```python
from build123d import *

# Parameters (mm, degrees)
MAIN_EXTRUSION_DEPTH    = 4
CORNER_LEAVE_R          = 5
D_GAGEMENT_M41_D        = 4.5
ESQUISSE4_W             = 22
ESQUISSE4_H             = 72
ENL_V_MAT_EXTRU_1_DEPTH = 4
ENL_V_MAT_EXTRU_2_DEPTH = 4
CONG_1_R                = 4


with BuildPart() as part:
    # Main scetch → Main extrusion (new body)
    with BuildSketch(Plane(origin=(0, 0, 0), x_dir=(1, 0, 0), z_dir=(0, 1, 0))):
        Polygon((-150, 0), (150, 0), (150, 175), (105, 220), (-105, 220), (-150, 175), align=None)
    extrude(amount=MAIN_EXTRUSION_DEPTH)

    # Corner leave
    corner_leave_edges = [part.edges().sort_by_distance(p)[0] for p in [
        (150, 2, 0),
        (-150, 2, 0),
        (-150, 2, -175),
        (-105, 2, -220),
        (105, 2, -220),
        (150, 2, -175),
    ]]
    fillet(corner_leave_edges, radius=CORNER_LEAVE_R)

    # Dégagement M41 (through all)
    with Locations(Plane(origin=(0, 4, 0), x_dir=(1, 0, 0), z_dir=(0, 1, 0))):
        with Locations((-142, 8), (-142, 170), (142, 170), (142, 8), (0, 8)):
            Hole(D_GAGEMENT_M41_D / 2)

    # Esquisse4 → Enlèv. mat.-Extru.1 (cut)
    with BuildSketch(Plane(origin=(0, 4, 0), x_dir=(1, 0, 0), z_dir=(0, 1, 0))):
        with Locations((139, 58)):
            Rectangle(ESQUISSE4_W, ESQUISSE4_H)
    extrude(amount=-ENL_V_MAT_EXTRU_1_DEPTH, mode=Mode.SUBTRACT)

    # Esquisse5 → Enlèv. mat.-Extru.2 (cut)
    with BuildSketch(Plane(origin=(0, 4, 0), x_dir=(1, 0, 0), z_dir=(0, 1, 0))):
        Polygon((36.3, 200), (53, 200), (53, 220), (-4, 220), (-4, 200), align=None)
    extrude(amount=-ENL_V_MAT_EXTRU_2_DEPTH, mode=Mode.SUBTRACT)

    # Congé1
    cong_1_edges = [part.edges().sort_by_distance(p)[0] for p in [
        (150, 2, -94),
        (150, 2, -22),
        (128, 2, -22),
        (128, 2, -94),
        (53, 2, -220),
        (53, 2, -200),
        (-4, 2, -200),
        (-4, 2, -220),
    ]]
    fillet(cong_1_edges, radius=CONG_1_R)


solid = part.part
```
For this review, take the finished solid that the model builds, in its own axes (mm). Give positions to 0.01 mm unless a question says otherwise; leave off trailing zeros. Loops run counter-clockwise (first coordinate to the right, second up) from the corner with the lowest first, then second, coordinate; pieces in that order, holes last. Notation, with made-up numbers: M 5,21 L 25,21 A28 cw 25,55 Z; hole C -12,85.5 d3. An arc over 180 degrees is marked long. One line per item, written item: value. Start each with the question number.
Q1. For L1, parallel to X at y = 0.9, z = -170; L2, parallel to Z at x = 142, y = 0.85; L3, parallel to Z at x = -142, y = 2.5, list the stretches that pass through material, from the lowest coordinate up.
Q2. Clearance check with flat-ended pins moving along their axes: pin 1 Ø2 at (y, z) = (2.5, -209) entering from +X; pin 2 Ø1.2 at (x, y) = (141, 2.5) entering from -Z; pin 3 Ø1.2 at (x, y) = (24, 2) entering from -Z. State where each tip first meets the part, or that it passes through.
Q3. Add section B-B (x = -118.5). Give the boundary of the cut face in (y, z), and give its area (3 significant figures).
Q4. Add section A-A (y = 2.4). Count the separate pieces of the cut face and the enclosed holes in it, and give its area (3 significant figures).
Reply:
1. L1: -150 to -144.25, -139.75 to 139.75, 144.25 to 150
1. L2: -183 to -172.25, -167.75 to -94, -22 to -10.25, -5.75 to 0
1. L3: -183 to -172.25, -167.75 to -10.25, -5.75 to 0
2. pin 1: x = 117
2. pin 2: z = -184.6
2. pin 3: z = -200
3. outline: M 0,-206.5 L 4,-206.5 L 4,0 L 0,0 Z
3. area: 826 mm²
4. separate pieces: 1
4. enclosed holes: 5
4. area: 61,200 mm²
